```python
from build123d import *

# Parameters (mm, degrees)
SKETCH_2_R      = 1.5
EXTRUDE_1_DEPTH = 1.25
FILLET_1_R      = 2.7


with BuildPart() as part:
    # 草图2 → 凸台-拉伸1 (new, symmetric)
    with BuildSketch(Plane.XY):
        with BuildLine():
            Line((7.33426448, -37.414752853), (7.5, -34.008214709))
            ThreePointArc((7.5, -34.008214709), (0, 39.35), (-7.5, -34.008214709))
            Line((-7.5, -34.008214709), (-7.33426448, -37.414752853))
            ThreePointArc((-7.33426448, -37.414752853), (-6.588395249, -39.252616986), (-4.858753275, -40.223391997))
            Line((-4.858753275, -40.223391997), (-1.5, -40.815630821))
            Line((-1.5, -40.815630821), (-1.5, -32.715630821))
            ThreePointArc((-1.5, -32.715630821), (0, 32.75), (1.5, -32.715630821))
            Line((1.5, -32.715630821), (1.5, -40.815630821))
            Line((1.5, -40.815630821), (4.858753275, -40.223391997))
            ThreePointArc((4.858753275, -40.223391997), (6.588395249, -39.252616986), (7.33426448, -37.414752853))
        make_face()
        with Locations((4.5, -36.523827839)):
            Circle(SKETCH_2_R, mode=Mode.SUBTRACT)
        with Locations(Location((-4.5, -36.523827839, 0), (0, 0, 180))):
            Circle(SKETCH_2_R, mode=Mode.SUBTRACT)
    extrude(amount=EXTRUDE_1_DEPTH, both=True)

    # 圆角1
    fillet_1_edges = [part.edges().sort_by_distance(p)[0] for p in [
        (-7.5, -34.008214709, 0),
        (7.5, -34.008214709, 0),
    ]]
    fillet(fillet_1_edges, radius=FILLET_1_R)


solid = part.part
```
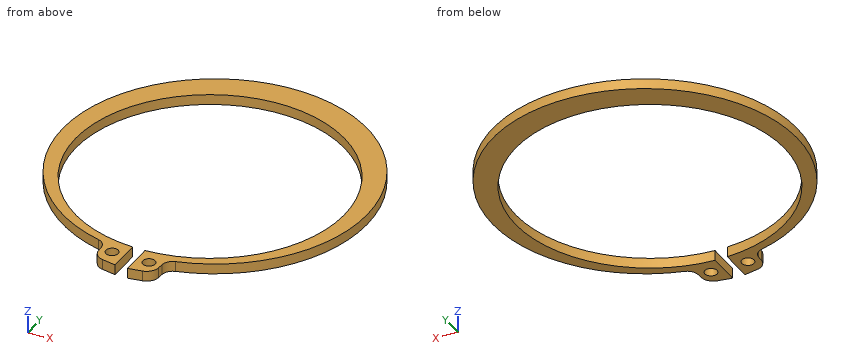
Could you check a few things on this model? Use its own coordinates, in mm. Coordinates: 2 decimals unless noted, no trailing zeros. Write each loop counter-clockwise with the first axis right and the second up, starting at its lowest first coordinate (ties: lowest second). Pieces come first, ordered by that corner, then holes. Notation, with made-up numbers: (-27.5, 23.5) - (11.5, 23.5) arc R12 cw to (11.5, 39.5) - close; hole circle Ø6 at (67, -16). An arc over 180 degrees is marked (long way). Use a Markdown table: item, result.
Q1. Imagine slicing it at C-C (z = 0.7). Count the separate pieces of the cut face and the enclosed holes in it, and give its area (3 significant figures).
Geometry check:
| item | result |
|---|---|
| separate pieces | 1 |
| enclosed holes | 2 |
| area | 993 mm2 |
Q2. Imagine slicing it at B-B (x = -26). List the corners of the cut face in (y, z) for me, and give its area (3 significant figures).
Geometry check:
| item | result |
|---|---|
| outline | (-24.13, -1.25) - (-19.91, -1.25) - (-19.91, 1.25) - (-24.13, 1.25) - close; (19.91, -1.25) - (28.7, -1.25) - (28.7, 1.25) - (19.91, 1.25) - close |
| area | 32.5 mm2 |
Q3. I'm going to push flat-ended pins straight in: pin 1 Ø1.5 at (x, z) = (-14.5, 0.5) entering from +Y; pin 2 Ø0.8 at (y, z) = (-37, -0.5) entering from +X; pin 3 Ø0.8 at (y, z) = (-37, 0) entering from -X. Where does each tip first touch, or does it pass through?
Geometry check:
| item | result |
|---|---|
| pin 1 | stops at y = 36.71 |
| pin 2 | stops at x = 7.37 |
| pin 3 | stops at x = -7.37 |
Q4. Please list where these lines run through material, in increasing order: L1, parallel to Y at x = 4.5, z = -0.5; L2, parallel to X at y = -0.5, z = 0.55; L3, parallel to X at y = -19.5, z = -0.65.
Geometry check:
| item | result |
|---|---|
| L1 | y = -40.29 to -38.02, -35.02 to -32.44, 32.44 to 39.08 |
| L2 | x = -36.96 to -32.75, 32.75 to 36.96 |
| L3 | x = -29.98 to -26.31, 26.31 to 29.98 |
Q5. Imagine slicing it at A-A (y = -28). List the corners of the cut face in (x, z) for me.
Geometry check:
| item | result |
|---|---|
| outline | (-21.36, -1.25) - (-16.99, -1.25) - (-16.99, 1.25) - (-21.36, 1.25) - close; (16.99, -1.25) - (21.36, -1.25) - (21.36, 1.25) - (16.99, 1.25) - close |
Q6. Imagine slicing it at D-D (x = 0). List the corners of the cut face in (y, z) for me.
Geometry check:
| item | result |
|---|---|
| outline | (32.75, -1.25) - (39.35, -1.25) - (39.35, 1.25) - (32.75, 1.25) - close |
